Autodesk Inventor part; units mm, degrees
ref_plane "YZ Plane" through (0, 0, 0) normal (1, 0, 0) x (0, 1, 0)
ref_plane "XZ Plane" through (0, 0, 0) normal (0, 1, 0) x (-1, 0, 0)
ref_plane "XY Plane" through (0, 0, 0) normal (0, 0, 1) x (1, 0, 0)
sketch "Sketch1" plane through (0, 0, 0) normal (0, 0, 1) x (1, 0, 0)
  line L0 (-28.8544, -12.7) -> (-28.8544, -28.8544)
  line L1 (-28.8544, -28.8544) -> (-12.7, -28.8544)
  line L2 (-12.7, -28.8544) -> (-12.7, -31.75)
  line L3 (-12.7, -31.75) -> (12.7, -31.75)
  line L4 (12.7, -31.75) -> (12.7, -28.8544)
  line L5 (12.7, -28.8544) -> (28.8544, -28.8544)
  line L6 (28.8544, -28.8544) -> (28.8544, -12.7)
  line L7 (28.8544, -12.7) -> (31.75, -12.7)
  line L8 (31.75, -12.7) -> (31.75, 12.7)
  line L9 (31.75, 12.7) -> (28.8544, 12.7)
  line L10 (28.8544, 12.7) -> (28.8544, 28.8544)
  line L11 (28.8544, 28.8544) -> (12.7, 28.8544)
  line L12 (12.7, 28.8544) -> (12.7, 31.75)
  line L13 (12.7, 31.75) -> (-12.7, 31.75)
  line L14 (-12.7, 31.75) -> (-12.7, 28.8544)
  line L15 (-12.7, 28.8544) -> (-28.8544, 28.8544)
  line L16 (-28.8544, 28.8544) -> (-28.8544, 12.7)
  line L17 (-28.8544, 12.7) -> (-31.75, 12.7)
  line L18 (-31.75, 12.7) -> (-31.75, -12.7)
  line L19 (-31.75, -12.7) -> (-28.8544, -12.7)
  point P0 (0, 0)
extrude "Extrusion1" add sketch "Sketch1" along normal blind 2.8956
properties part number "outside_box_front_back" material "Polycarbonate, Clear"
Can you work these out from the model? Positions are in its coordinate system, mm. A direction names the side the tool comes from. Give positions to 0.01 mm unless a question says otherwise; leave off trailing zeros. Loops run counter-clockwise (first coordinate to the right, second up) from the corner with the lowest first, then second, coordinate; pieces in that order, holes last. Notation, with made-up numbers: (9, 77) - (17, 77) arc R14 ccw to (17, 104) - close; hole circle Ø2 at (7.25, -11). An arc over 180 degrees is marked (long way). Return JSON: item names as keys, results as strings.
1. For faces 1 (the face through (-12.7, 30, 1)), 2 (the face through (21, 28.854, 1)), 3 (the face through (30, -12.7, 1)), which set-ups out of +Z, -Z, +X, -X, +Y, -Y let a thin tool reach every point of the face, with its end or its side?
Output values:
{"face 1": "+Z, -Z, -X, +Y", "face 2": "+Z, -Z, +X, +Y", "face 3": "+Z, -Z, +X, -Y"}
2. I'm going to push flat-ended pins straight in: pin 1 Ø0.9 at (x, z) = (30.5, 1.5) entering from +Y; pin 2 Ø0.9 at (y, z) = (24, 2) entering from +X; pin 3 Ø1.4 at (x, z) = (-21, 2) entering from -Y. Where does each tip first touch, or does it pass through?
Output values:
{"pin 1": "stops at y = 12.7", "pin 2": "stops at x = 28.85", "pin 3": "stops at y = -28.85"}
3. I want a section at B-B on x = 27.5. Please give me the cut outline in (y, z), and give its area (3 significant figures).
Output values:
{"outline": "(-28.85, 0) - (28.85, 0) - (28.85, 2.9) - (-28.85, 2.9) - close", "area": "167 mm²"}
4. If I drill on line 1 (Y direction, x = -17, z = 0.65); line 2 (X direction, y = 29, z = 1.25), over which ranges is the centre line in solid material (lowest first)?
Output values:
{"line 1": "y = -28.85 to 28.85", "line 2": "x = -12.7 to 12.7"}
5. I want a section at A-A on z = 2.2. Please give me the cut outline in (x, y), and give its area (3 significant figures).
Output values:
{"outline": "(-31.75, -12.7) - (-28.85, -12.7) - (-28.85, -28.85) - (-12.7, -28.85) - (-12.7, -31.75) - (12.7, -31.75) - (12.7, -28.85) - (28.85, -28.85) - (28.85, -12.7) - (31.75, -12.7) - (31.75, 12.7) - (28.85, 12.7) - (28.85, 28.85) - (12.7, 28.85) - (12.7, 31.75) - (-12.7, 31.75) - (-12.7, 28.85) - (-28.85, 28.85) - (-28.85, 12.7) - (-31.75, 12.7) - close", "area": "3,620 mm²"}
